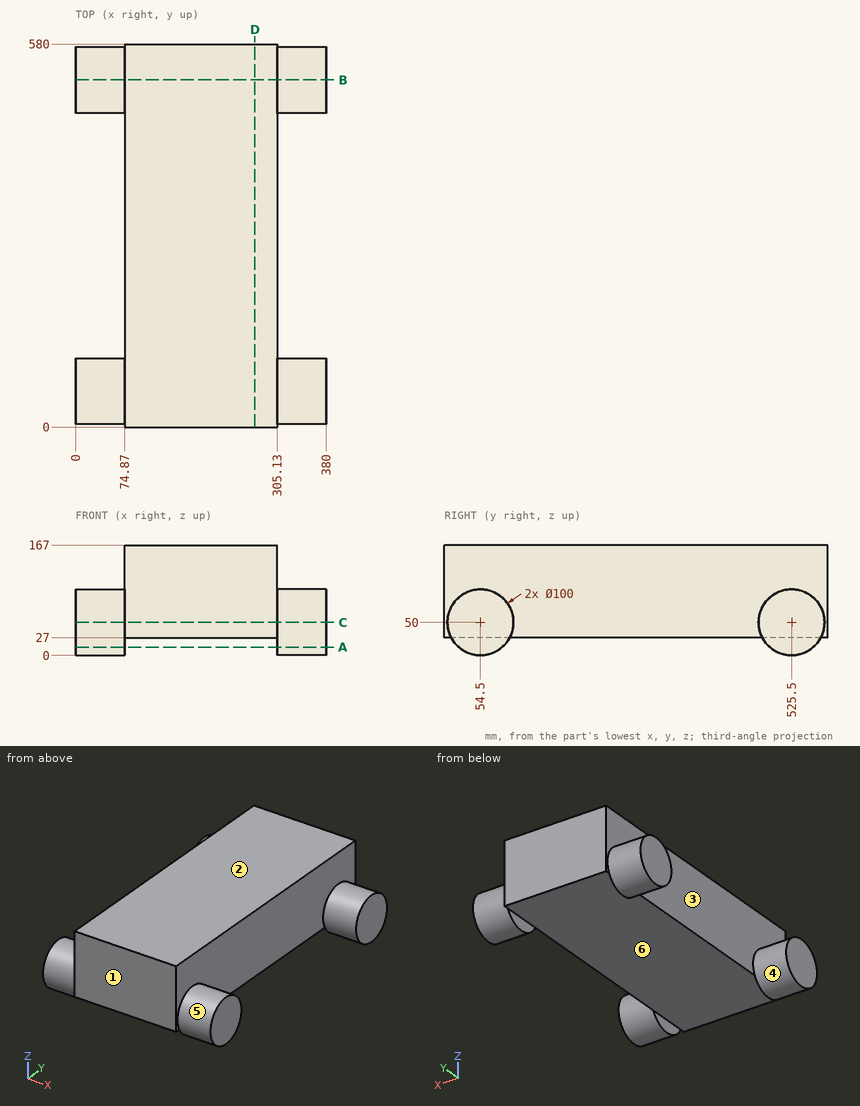
Check sheet for the drawn part. Datum: minimum x, y, z corner. Units: mm. A direction names the side the tool comes from. Coordinates: 2 decimals unless noted, no trailing zeros. Order: outer loops, then holes, each group sorted by start corner. A loop starts at its lowest first (then second) coordinate and runs counter-clockwise, first axis right, second up. Notation, with made-up numbers: (65.5, 26.5) - (88.5, 26.5) arc R18 ccw to (88.5, 33.5) - close; hole circle Ø3 at (76.25, 54.25). An arc over 180 degrees is marked (long way). Return JSON: item names as keys, results as strings.
(1) Mould release check, pull along Y, two halves, no side actions. Record for the marked faces 1, 2 and 3: pulls with the +Y half, pulls with the -Y half, needs draft (parallel to the pull), parting line crosses it, or undercut.
Filled sheet:
{"face 1": "pulls with the -Y half", "face 2": "needs draft", "face 3": "undercut"}
(2) Access from +Z, -Z, +X, -X, +Y, -Y to the whole of each face (thin tool, end or side, straight path). Record for the marked faces 4, 5 and 6.
Filled sheet:
{"face 4": "-X", "face 5": "+X", "face 6": "-Z, +Y, -Y"}
(3) Go/stop test with flat-tipped pins: pin 1 (12 mm diameter, centred on x = 112.5, y = 305, fed in from -Z); pin 2 (3 mm diameter, centred on y = 358, z = 74, fed in from -X); pin 3 (5 mm diameter, centred on y = 334, z = 84.5, fed in from +X). Record where each tip stops, or that it passes through.
Filled sheet:
{"pin 1": "stops at z = 27", "pin 2": "stops at x = 74.87", "pin 3": "stops at x = 305.13"}
(4) Thickness scan on line 1 along X through (y, z) = (239, 79); line 2 along Z through (x, y) = (80.5, 328); line 3 along Y through (x, z) = (36.5, 88). Record the ranges inside material, lowest first.
Filled sheet:
{"line 1": "x = 74.87 to 305.13", "line 2": "z = 27 to 167", "line 3": "y = 22 to 87, 493 to 558"}
(5) Section check A-A, the plane z = 12.5. Record the cut outline in (x, y), and give its area (3 significant figures).
Filled sheet:
{"outline": "(0, 21.43) - (74.87, 21.43) - (74.87, 87.57) - (0, 87.57) - close; (0, 492.43) - (74.87, 492.43) - (74.87, 558.57) - (0, 558.57) - close; (305.13, 21.43) - (380, 21.43) - (380, 87.57) - (305.13, 87.57) - close; (305.13, 492.43) - (380, 492.43) - (380, 558.57) - (305.13, 558.57) - close", "area": "19,800 mm^2"}
(6) Section check D-D, the plane x = 271.5. Record the cut outline in (y, z).
Filled sheet:
{"outline": "(0, 27) - (580, 27) - (580, 167) - (0, 167) - close"}
(7) Section check C-C, the plane z = 50. Record the cut outline in (x, y), and give its area (3 significant figures).
Filled sheet:
{"outline": "(0, 4.5) - (74.87, 4.5) - (74.87, 0) - (305.13, 0) - (305.13, 4.5) - (380, 4.5) - (380, 104.5) - (305.13, 104.5) - (305.13, 475.5) - (380, 475.5) - (380, 575.5) - (305.13, 575.5) - (305.13, 580) - (74.87, 580) - (74.87, 575.5) - (0, 575.5) - (0, 475.5) - (74.87, 475.5) - (74.87, 104.5) - (0, 104.5) - close", "area": "163,000 mm^2"}
(8) Section check B-B, the plane y = 525.5. Record the cut outline in (x, z).
Filled sheet:
{"outline": "(0, 0) - (74.87, 0) - (74.87, 27) - (305.13, 27) - (305.13, 0) - (380, 0) - (380, 100) - (305.13, 100) - (305.13, 167) - (74.87, 167) - (74.87, 100) - (0, 100) - close"}
